Read the model definition and answer for the solid it produces. Units are mm, in the model's axes. A direction names the side the tool comes from. Coordinates: 2 decimals unless noted, no trailing zeros. Write each loop counter-clockwise with the first axis right and the second up, starting at its lowest first coordinate (ties: lowest second). Pieces come first, ordered by that corner, then holes. Notation, with made-up numbers: (15, 43.25) -> (71, 43.25) arc R23 cw to (71, 71.25) -> close; hole circle Ø2 at (22, 24). An arc over 180 degrees is marked (long way). One line per item, written item: value. Start each with the question number.
1. For a pull along X with two mould halves and no side action, classify faces 1 (the flat face through (15.75, 40, 0)), 2 (the flat face through (-23, 50.25, 0)), 3 (the cylindrical face through (41.776, 28.128, -0.021)) as pulls with the +X half, pulls with the -X half, needs draft (parallel to the pull), parting line crosses it, or undercut.
2. Find section A-A, the plane x = 0. Write down the section's boundary in (y, z).
3. For faces 4 (the flat face through (-11.25, 40, 0)), 5 (the cylindrical face through (-12.52, 33.75, 0.02)), 6 (the flat face through (-26.5, -20, 0)), determine the directions among +Z, -Z, +X, -X, +Y, -Y from which every point of the face is accessible in a straight line to the end or side of a thin tool.
4. Find section C-C, the plane z = 0.15. State how many separate pieces and enclosed holes the cut face has, and give its area (3 significant figures).
5. Consider line 1 along X through (y, z) = (47, -1.3); line 2 along X through (y, z) = (32.5, -1.1); line 3 along Y through (x, z) = (0, 0.7). Determine where each line is inside the solid, lowest interval first.
6. Given P1, Ø0.9, axis at y = -20, z = 0.5, coming from the -X side; P2, Ø0.9, axis at y = 44.5, z = 0.5, coming from the +X side; P3, Ø0.9, axis at y = 31.5, z = 0, coming from the -X side, each flat-ended and moving along its own axis, determine where each tip first touches the part or whether it passes through.
7. Find section B-B, the plane y = -16. Write down the section's boundary in (x, z), and give its area (3 significant figures).
```python
from build123d import *

# Parameters (mm, degrees)
SKETCH_1_W           = 53
SKETCH_1_H           = 54.5
SKETCH_1_R           = 23.5
EXTRUDE_1_DEPTH      = 1.5
SKETCH_2_R           = 1.65
SKETCH_2_R_2         = 2.15
CUT_EXTRUDE_1_DEPTH  = 3
FILLET_1_R           = 5
CUT_EXTRUDE_2_DEPTH  = 5
SKETCH_4_W           = 53
SKETCH_4_H           = 3
EXTRUDE_2_DEPTH      = 3
FILLET_2_R           = 2.5
SKETCH_5_W           = 50
SKETCH_5_H           = 20
EXTRUDE_3_DEPTH      = 3
CUT_EXTRUDE_9_DEPTH  = 3
FILLET_3_R           = 5
SKETCH_8_W           = 15
SKETCH_8_H           = 3
EXTRUDE_4_DEPTH      = 3
CUT_EXTRUDE_10_DEPTH = 3


with BuildPart() as part:
    # 草图1 → 凸台-拉伸1 (new, symmetric)
    with BuildSketch(Plane.XY):
        Rectangle(SKETCH_1_W, SKETCH_1_H)
        Circle(SKETCH_1_R, mode=Mode.SUBTRACT)
    extrude(amount=EXTRUDE_1_DEPTH, both=True)

    # 草图2 → 切除-拉伸1 (cut)
    with BuildSketch(Plane(origin=(0, 0, -1.5), x_dir=(-1, 0, 0), z_dir=(0, 0, -1))):
        with Locations((-21.5, -22.25)):
            Circle(SKETCH_2_R)
        with Locations((-21.213203436, 20.463203436)):
            Circle(SKETCH_2_R_2)
        with Locations((21.5, -22.25)):
            Circle(SKETCH_2_R)
        with Locations((21.213203436, 20.463203436)):
            Circle(SKETCH_2_R_2)
    extrude(amount=-CUT_EXTRUDE_1_DEPTH, mode=Mode.SUBTRACT)

    # 圆角1
    fillet_1_edges = [part.edges().sort_by_distance(p)[0] for p in [
        (26.5, -27.25, 0),
        (-26.5, -27.25, 0),
    ]]
    fillet(fillet_1_edges, radius=FILLET_1_R)

    # 草图3 → 切除-拉伸2 (cut)
    with BuildSketch(Plane.XY.offset(1.5)):
        Polygon((0, 0), (15.732794835, 27.25), (-15.732794835, 27.25), align=None)
    extrude(amount=-CUT_EXTRUDE_2_DEPTH, mode=Mode.SUBTRACT)

    # 草图4 → 凸台-拉伸2 (add)
    with BuildSketch(Plane(origin=(0, 27.25, 0), x_dir=(1, 0, 0), z_dir=(0, 1, 0))):
        Rectangle(SKETCH_4_W, SKETCH_4_H)
    extrude(amount=EXTRUDE_2_DEPTH)

    # 圆角2
    fillet_2_edges = [part.edges().sort_by_distance(p)[0] for p in [
        (11.75, 20.351596989, 0),
        (-11.75, 20.351596989, 0),
        (-15.732794835, 27.25, 0),
        (15.732794835, 27.25, 0),
    ]]
    fillet(fillet_2_edges, radius=FILLET_2_R)

    # 草图5 → 凸台-拉伸3 (add)
    with BuildSketch(Plane.XY.offset(1.5)):
        Polygon((-26.5, -17.25), (-45, 30.25), (-26.5, 30.25), align=None)
        Polygon((26.5, -17.25), (45, 30.25), (26.5, 30.25), align=None)
        with Locations((0, 40.25)):
            Rectangle(SKETCH_5_W, SKETCH_5_H)
    extrude(amount=-EXTRUDE_3_DEPTH)

    # 草图6 → 切除-拉伸9 (cut)
    with BuildSketch(Plane.XY.offset(1.5)):
        with BuildLine():
            Line((-11.177124344, 33.25), (-7.5, 33.25))
            Line((-7.5, 33.25), (-7.5, 30.25))
            Line((-7.5, 30.25), (-11.177124344, 30.25))
            ThreePointArc((-11.177124344, 30.25), (-12.5, 29.75), (-13.822875656, 30.25))
            Line((-13.822875656, 30.25), (-17.5, 30.25))
            Line((-17.5, 30.25), (-17.5, 33.25))
            Line((-17.5, 33.25), (-13.822875656, 33.25))
            ThreePointArc((-13.822875656, 33.25), (-12.5, 33.75), (-11.177124344, 33.25))
        make_face()
        with BuildLine():
            Line((13.822875656, 33.25), (17.5, 33.25))
            Line((17.5, 33.25), (17.5, 30.25))
            Line((17.5, 30.25), (13.822875656, 30.25))
            ThreePointArc((13.822875656, 30.25), (12.5, 29.75), (11.177124344, 30.25))
            Line((11.177124344, 30.25), (7.5, 30.25))
            Line((7.5, 30.25), (7.5, 33.25))
            Line((7.5, 33.25), (11.177124344, 33.25))
            ThreePointArc((11.177124344, 33.25), (12.5, 33.75), (13.822875656, 33.25))
        make_face()
    extrude(amount=-CUT_EXTRUDE_9_DEPTH, mode=Mode.SUBTRACT)

    # 圆角3
    fillet_3_edges = [part.edges().sort_by_distance(p)[0] for p in [
        (-45, 30.25, 0),
        (45, 30.25, 0),
    ]]
    fillet(fillet_3_edges, radius=FILLET_3_R)

    # 草图8 → 凸台-拉伸4 (add)
    with BuildSketch(Plane.XY.offset(1.5)):
        with Locations((-13.5, 51.75)):
            Rectangle(SKETCH_8_W, SKETCH_8_H)
        with Locations((13.5, 51.75)):
            Rectangle(SKETCH_8_W, SKETCH_8_H)
    extrude(amount=-EXTRUDE_4_DEPTH)

    # 草图9 → 切除-拉伸10 (cut)
    with BuildSketch(Plane.XY.offset(1.5)):
        Polygon((-15.75, 53.25), (-15.75, 47.25), (-17.75, 47.25), (-17.75, 42.25), (-15.75, 42.25), (-15.75, 38.25), (-11.25, 38.25), (-11.25, 42.25), (-9.25, 42.25), (-9.25, 47.25), (-11.25, 47.25), (-11.25, 53.25), align=None)
        Polygon((11.25, 47.25), (11.25, 53.25), (15.75, 53.25), (15.75, 47.25), (17.75, 47.25), (17.75, 42.25), (15.75, 42.25), (15.75, 38.25), (11.25, 38.25), (11.25, 42.25), (9.25, 42.25), (9.25, 47.25), align=None)
    extrude(amount=-CUT_EXTRUDE_10_DEPTH, mode=Mode.SUBTRACT)


solid = part.part
```
Answer block:
1. face 1: undercut
1. face 2: needs draft
1. face 3: pulls with the +X half
2. outline: (-27.25, -1.5) -> (-23.5, -1.5) -> (-23.5, 1.5) -> (-27.25, 1.5) -> close; (27.25, -1.5) -> (50.25, -1.5) -> (50.25, 1.5) -> (27.25, 1.5) -> close
3. face 4: +Z, -Z, +Y
3. face 5: +Z, -Z
3. face 6: +Z, -Z, -X, -Y
4. separate pieces: 1
4. enclosed holes: 7
4. area: 2,830 mm2
5. line 1: x = -25 to -17.75, -9.25 to 9.25, 17.75 to 25
5. line 2: x = -25 to -17.5, -7.5 to 7.5, 17.5 to 25
5. line 3: y = -27.25 to -23.5, 27.25 to 50.25
6. P1: stops at x = -26.5
6. P2: stops at x = 25
6. P3: stops at x = -25
7. outline: (-26.99, -1.5) -> (-17.21, -1.5) -> (-17.21, 1.5) -> (-26.99, 1.5) -> close; (17.21, -1.5) -> (26.99, -1.5) -> (26.99, 1.5) -> (17.21, 1.5) -> close
7. area: 58.6 mm2
